Geometry check sheet. Reference: drawing and pictorial views, mm from the part's lowest x, y, z. Give positions to 0.01 mm unless a question says otherwise; leave off trailing zeros. Order: outer loops, then holes, each group sorted by start corner. A loop starts at its lowest first (then second) coordinate and runs counter-clockwise, first axis right, second up. Notation, with made-up numbers: M -9,12 L 47,12 A22 cw 47,37 Z; hole C 68,57 d2. An arc over 180 degrees is marked long. Answer as CSV lines item,"result".
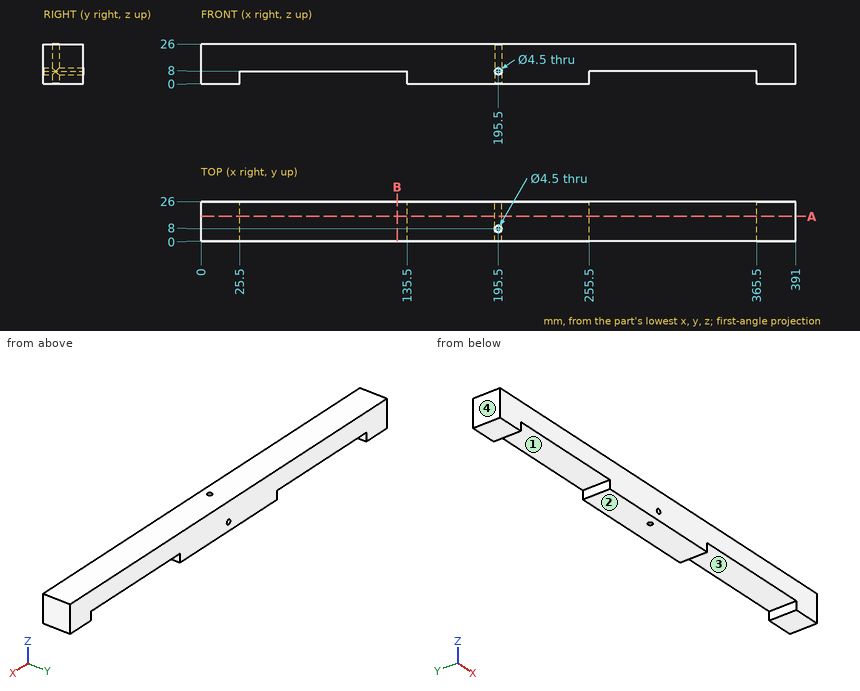
(1) Gauge pin test, flat end, axial feed: P1, Ø12, axis at x = 269.5, y = 10.5, coming from the -Z side. Record the tip position at first contact, or that the pin passes through.
The answers:
P1,"stops at z = 8"
(2) Section check B-B on x = 129. Enter the section's corners in (y, z).
The answers:
outline,"M 0,8 L 26,8 L 26,26 L 0,26 Z"
(3) Draft check along X on the marked faces 1, 2, 3 and 4. Enter one of: +X half, -X half, draft (parallel to the pull), parting line (faces both ways), or undercut.
The answers:
face 1,"undercut"
face 2,"draft"
face 3,"undercut"
face 4,"-X half"
(4) Section check A-A on y = 16.25. Enter the section's corners in (x, z), then the cut area to 3 significant figures.
The answers:
outline,"M 0,0 L 25.5,0 L 25.5,8 L 135.5,8 L 135.5,0 L 255.5,0 L 255.5,8 L 365.5,8 L 365.5,0 L 391,0 L 391,26 L 0,26 Z; hole C 195.5,8 d4.5"
area,"8,390 mm2"
(5) Material ranges on line 1 (X direction, y = 8.5, z = 12); line 2 (Y direction, x = 195.5, z = 18), recorded low to high.
The answers:
line 1,"x = 0 to 193.31, 197.69 to 391"
line 2,"y = 0 to 5.75, 10.25 to 26"
